The listing builds one solid part. Answer for the finished solid, in the listing's coordinates (mm). Round coordinates to 2 decimals unless told otherwise and drop trailing zeros. Write each loop counter-clockwise with the first axis right and the second up, starting at its lowest first coordinate (ties: lowest second). Pieces come first, ordered by that corner, then holes.
Autodesk Inventor part; units mm, degrees
ref_plane "YZ Plane" through (0, 0, 0) normal (1, 0, 0) x (0, 1, 0)
ref_plane "XZ Plane" through (0, 0, 0) normal (0, 1, 0) x (-1, 0, 0)
ref_plane "XY Plane" through (0, 0, 0) normal (0, 0, 1) x (1, 0, 0)
ref_plane "Płaszczyzna konstrukcyjna1" through (0, 0.1, -1.5872) normal (0, 1, 0) x (1, 0, 0)
sketch "Szkic3" plane through (0, 0.1, -1.5872) normal (0, 1, 0) x (1, 0, 0)
  line L0 (6, 4.5) -> (-6, 4.5)
  line L1 (-6, 4.5) -> (-6, -4.5)
  line L2 (-6, -4.5) -> (6, -4.5)
  line L3 (6, -4.5) -> (6, 4.5)
  line L4 (9.543, 0) -> (-12.3472, 0)
  line L5 (0, 10.0787) -> (0, -13.253)
  line L6 (6, 4.5) -> (11.25, 4.5)
  line L7 (13.25, 2.5) -> (13.25, -2.5)
  line L8 (11.25, -4.5) -> (6, -4.5)
  line L9 (6, -4.5) -> (6, 4.5)
  arc A0 (13.25, 2.5) -> (11.25, 4.5) centre (11.25, 2.5) ccw
  arc A1 (11.25, -4.5) -> (13.25, -2.5) centre (11.25, -2.5) ccw
  line L10 (-13.25, 2.5) -> (-13.25, -2.5)
  arc A2 (-11.25, 4.5) -> (-13.25, 2.5) centre (-11.25, 2.5) ccw
  line L11 (-6, 4.5) -> (-11.25, 4.5)
  arc A3 (-13.25, -2.5) -> (-11.25, -4.5) centre (-11.25, -2.5) ccw
  line L12 (-11.25, -4.5) -> (-6, -4.5)
  line L13 (-13.25, 0.45) -> (-9, 0.45)
  circle A4 centre (9.543, 0) radius 1.75
  circle A5 centre (-9.543, 0) radius 1.75
  point P0 (0, 0)
  point P1 (13.25, 4.5)
  dimension "d26" = 12
  dimension "d25" = 9
  dimension "d24" = 4.5
  dimension "d23" = 6
  dimension "d22" = 7.25
  dimension "d20" = 2
  dimension "d19" = 4.25
  dimension "d18" = 4.05
  dimension "d16" = 19.086
  dimension "d21" = 3.707
  dimension "d17" = 3.5
  dimension "d15" = 3.5
extrude "Wyciągnięcie proste3" add sketch "Szkic3" along normal blind 1 contours L3 L4 L5 L0 | L6 A0 L7 A1 L8 L3 | L5 L4 L1 L0 | L3 L2 L5 L4 | L1 L4 A5 L13 L10 A2 L11 | L5 L2 L1 L4 | L1 L12 A3 L10 L13 A5 L4
properties part number "prent1"
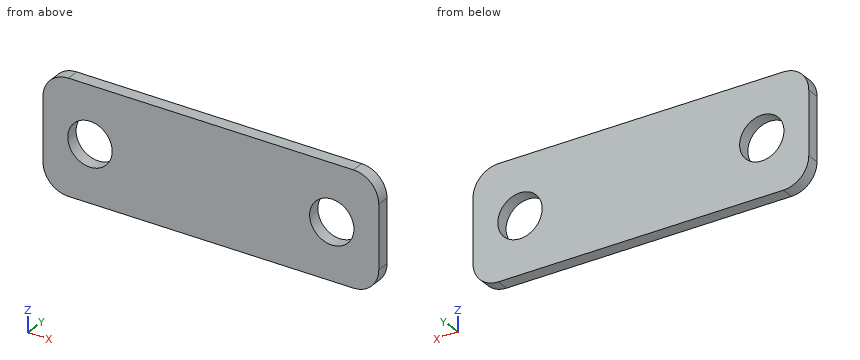
1. Section A-A on z = -0.5 is taken. Determine the outline of the cut face in (x, y), plus the area to 3 significant figures.
Geometry says:
outline: (-13.25, 0.1) - (-10.91, 0.1) - (-10.91, 1.1) - (-13.25, 1.1) - close; (-8.17, 0.1) - (8.17, 0.1) - (8.17, 1.1) - (-8.17, 1.1) - close; (10.91, 0.1) - (13.25, 0.1) - (13.25, 1.1) - (10.91, 1.1) - close
area: 21.0 mm2
2. Given pin 1 (3 mm diameter, centred on x = -9.54, z = -1.59, fed in from +Y), flat-ended and moving along its own axis, determine where the tip first touches the part or whether it passes through.
Geometry says:
pin 1: passes through
3. Straight lines are drawn through the part: line 1 along X through (y, z) = (0.65, -1.5); line 2 along X through (y, z) = (0.7, -1); line 3 along Z through (x, y) = (-10, 0.4). For each, find the intervals that lie inside material, in ascending order.
Geometry says:
line 1: x = -13.25 to -11.29, -7.8 to 7.8, 11.29 to 13.25
line 2: x = -13.25 to -11.19, -7.89 to 7.89, 11.19 to 13.25
line 3: z = -6.09 to -3.28, 0.1 to 2.91
4. Section C-C on x = 9.5 is taken. Determine the outline of the cut face in (y, z).
Geometry says:
outline: (0.1, -6.09) - (1.1, -6.09) - (1.1, -3.34) - (0.1, -3.34) - close; (0.1, 0.16) - (1.1, 0.16) - (1.1, 2.91) - (0.1, 2.91) - close
5. Section B-B on y = 0.8 is taken. Determine the outline of the cut face in (x, z).
Geometry says:
outline: (-13.25, -4.09) arc R2 ccw to (-11.25, -6.09) - (11.25, -6.09) arc R2 ccw to (13.25, -4.09) - (13.25, 0.91) arc R2 ccw to (11.25, 2.91) - (-11.25, 2.91) arc R2 ccw to (-13.25, 0.91) - close; hole circle Ø3.5 at (-9.54, -1.59); hole circle Ø3.5 at (9.54, -1.59)
